Answer from the drawing. Dimensions are ordinates in mm from the lowest x, y and z of the part. A direction names the side the tool comes from. Give positions to 0.01 mm unless a question says otherwise; leave off trailing zeros. Order: outer loops, then holes, each group sorted by start corner. A loop starts at its lowest first (then second) coordinate and runs counter-clockwise, first axis right, second up. Notation, with made-up numbers: (74, -20) -> (110, -20) arc R24 cw to (110, 9) -> close; hole circle Ø1 at (37, 24.5). An arc over 180 degrees is marked (long way). One line per question, with ' | ' between items. Start each with the question number.
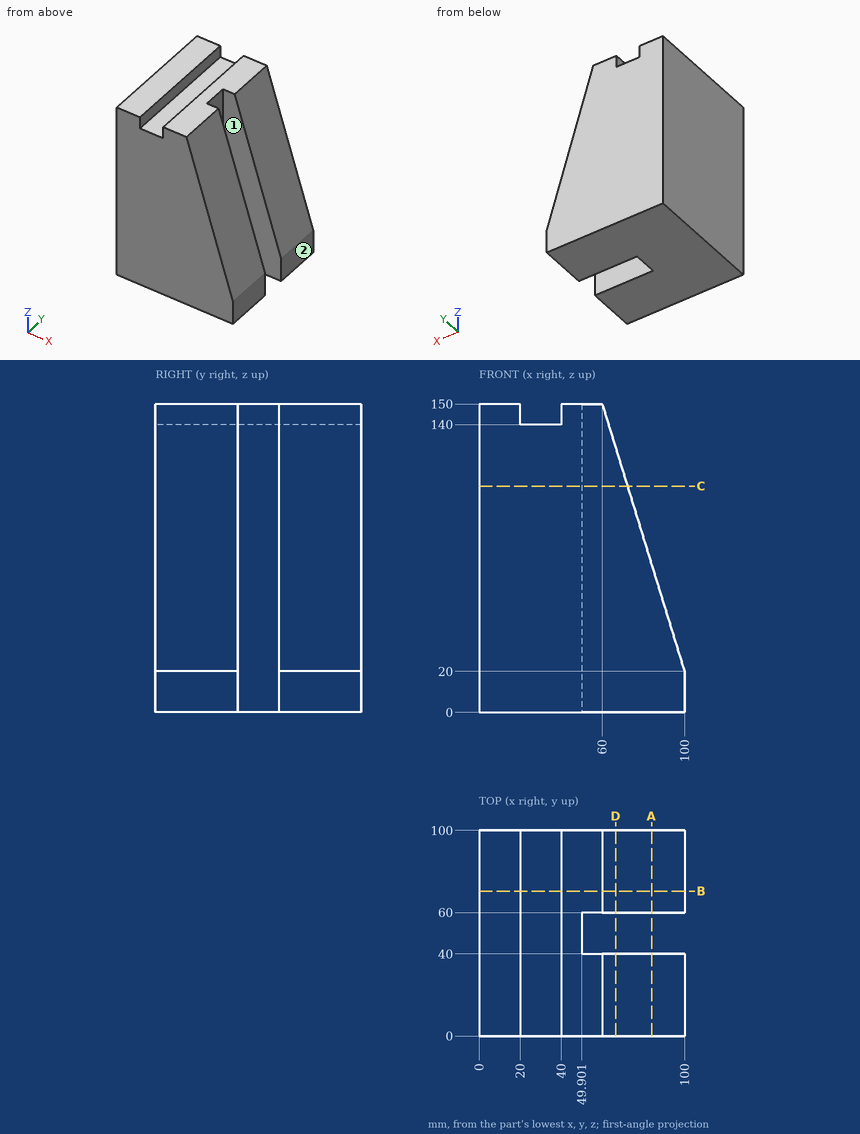
(1) The part is cut by section C-C on z = 110. Determine the outline of the cut face in (x, y).
(2) The part is cut by section D-D on x = 66.5. Determine the outline of the cut face in (y, z) (1 decimal).
(3) Given P1, Ø2, axis at y = 16, z = 120.5, coming from the +X side (1 decimal); P2, Ø1, axis at y = 88.5, z = 22, coming from the +X side; P3, Ø6, axis at y = 53.5, z = 48.5, coming from the +X side; P4, Ø5, axis at x = 70, z = 128, coming from the +Y side, each flat-ended and moving along its own axis, determine where each tip first touches the part or whether it passes through.
(4) For the marked faces 1 and 2, determine the directions among +Z, -Z, +X, -X, +Y, -Y from which every point of the face is accessible in a straight line to the end or side of a thin tool.
(5) The part is cut by section B-B on y = 70.5. Determine the outline of the cut face in (x, z), plus the area to 3 significant figures.
(6) The part is cut by section A-A on x = 84. Determine the outline of the cut face in (y, z), plus the area to 3 significant figures.
(7) Consider line 1 (Y direction, x = 87, z = 55.5); line 2 (Z direction, x = 29, y = 70); line 3 (X direction, y = 46, z = 30). Determine where each line is inside the solid, lowest interval first.
Result sheet:
1) outline: (0, 0) -> (72.31, 0) -> (72.31, 40) -> (49.9, 40) -> (49.9, 60) -> (72.31, 60) -> (72.31, 100) -> (0, 100) -> close
2) outline: (0, 0) -> (40, 0) -> (40, 128.9) -> (0, 128.9) -> close; (60, 0) -> (100, 0) -> (100, 128.9) -> (60, 128.9) -> close
3) P1: stops at x = 69.4 | P2: stops at x = 99.54 | P3: stops at x = 49.9 | P4: passes through
4) face 1: +Z, -Z, +X | face 2: +Z, -Z, +X, +Y, -Y
5) outline: (0, 0) -> (100, 0) -> (100, 20) -> (60, 150) -> (40, 150) -> (40, 140) -> (20, 140) -> (20, 150) -> (0, 150) -> close | area: 12,200 mm^2
6) outline: (0, 0) -> (40, 0) -> (40, 72) -> (0, 72) -> close; (60, 0) -> (100, 0) -> (100, 72) -> (60, 72) -> close | area: 5,760 mm^2
7) line 1: y = 0 to 40, 60 to 100 | line 2: z = 0 to 140 | line 3: x = 0 to 49.9
